```python
from build123d import *

# Parameters (mm, degrees)
SKETCH1_W                      = 20
SKETCH1_H                      = 8.2
BOSS_EXTRUDE1_DEPTH            = 21
SKETCH2_W                      = 8.2
SKETCH2_H                      = 0.8
BOSS_EXTRUDE2_DEPTH            = 5
SKETCH3_W                      = 8.2
SKETCH3_H                      = 0.8
BOSS_EXTRUDE3_DEPTH            = 5
CUT_EXTRUDE1_REACH             = 35.664
CUT_EXTRUDE2_REACH             = 33.217
F_2_0_2_DIAMETER_HOLE1_D       = 2
BOSS_EXTRUDE6_DEPTH            = 3
CUT_EXTRUDE4_REACH             = 36.986
SKETCH12_W                     = 6.2
SKETCH12_H                     = 2
BOSS_EXTRUDE7_DEPTH            = 3.5
BOSS_EXTRUDE7_TAPER            = 8
SKETCH15_R                     = 2
CUT_EXTRUDE5_DEPTH             = 5
SKETCH17_R                     = 3
SKETCH17_R_2                   = 2
BOSS_EXTRUDE10_DEPTH           = 0.2
BOSS_EXTRUDE10_DRAFT           = 45
SKETCH17_R_3                   = 1
BOSS_EXTRUDE10_PROFILE_2_DEPTH = 0.2
BOSS_EXTRUDE10_PROFILE_2_DRAFT = 45


with BuildPart() as part:
    # Sketch1 → Boss-Extrude1 (new body)
    with BuildSketch(Plane(origin=(0, 0, 0), x_dir=(1, 0, 0), z_dir=(0, 1, 0))):
        with Locations((10, -4.1)):
            Rectangle(SKETCH1_W, SKETCH1_H)
    extrude(amount=BOSS_EXTRUDE1_DEPTH)

    # Sketch2 → Boss-Extrude2 (add)
    with BuildSketch(Plane(origin=(20, 0, 0), x_dir=(0, 0, -1), z_dir=(1, 0, 0))):
        with Locations((-4.1, 16.4)):
            Rectangle(SKETCH2_W, SKETCH2_H)
    extrude(amount=BOSS_EXTRUDE2_DEPTH)

    # Sketch3 → Boss-Extrude3 (add)
    with BuildSketch(Plane.ZY):
        with Locations((4.1, 16.4)):
            Rectangle(SKETCH3_W, SKETCH3_H)
    extrude(amount=BOSS_EXTRUDE3_DEPTH)

    # Sketch4 → Cut-Extrude1 (cut, up to next)
    with BuildSketch(Plane.XY.offset(8.2), mode=Mode.PRIVATE) as cut_extrude1_sk1:
        Polygon((20, 19), (15, 21), (20, 21), align=None)
    cut_extrude1_tool1 = extrude(cut_extrude1_sk1.sketch, amount=-CUT_EXTRUDE1_REACH, mode=Mode.PRIVATE) & part.part
    add(cut_extrude1_tool1.solids().sort_by_distance((18.333333, 20.333333, 8.2))[0], mode=Mode.SUBTRACT)

    # Sketch8 → Cut-Extrude2 (cut, up to next)
    with BuildSketch(Plane(origin=(0, 16.8, 0), x_dir=(1, 0, 0), z_dir=(0, 1, 0)), mode=Mode.PRIVATE) as cut_extrude2_sk1:
        with BuildLine():
            Line((-5, 0), (0, 0))
            ThreePointArc((0, 0), (-4.1, -4.1), (0, -8.2))
            Line((0, -8.2), (-5, -8.2))
            Line((-5, -8.2), (-5, 0))
        make_face()
    cut_extrude2_tool1 = extrude(cut_extrude2_sk1.sketch, amount=-CUT_EXTRUDE2_REACH, mode=Mode.PRIVATE) & part.part
    # Sketch8 → Cut-Extrude2 (cut, up to next)
    with BuildSketch(Plane(origin=(0, 16.8, 0), x_dir=(1, 0, 0), z_dir=(0, 1, 0)), mode=Mode.PRIVATE) as cut_extrude2_sk2:
        with BuildLine():
            Line((20, -8.2), (25, -8.2))
            Line((25, -8.2), (25, 0))
            Line((25, 0), (20, 0))
            ThreePointArc((20, 0), (24.1, -4.1), (20, -8.2))
        make_face()
    cut_extrude2_tool2 = extrude(cut_extrude2_sk2.sketch, amount=-CUT_EXTRUDE2_REACH, mode=Mode.PRIVATE) & part.part
    add(cut_extrude2_tool1.solids().sort_by_distance((-2.5, 16.8, 8.103958))[0], mode=Mode.SUBTRACT)
    add(cut_extrude2_tool2.solids().sort_by_distance((24.196042, 16.8, 4.1))[0], mode=Mode.SUBTRACT)

    # Ø2.0 (2) Diameter Hole1 (through all)
    with Locations(Plane(origin=(-2.05, 16.8, 4.1), x_dir=(0, 0, 1), z_dir=(0, 1, 0))):
        with Locations((0, 0), (0, 24.1)):
            Hole(F_2_0_2_DIAMETER_HOLE1_D / 2)

    # Sketch10 → Boss-Extrude6 (add)
    with BuildSketch(Plane(origin=(0, 21, 0), x_dir=(1, 0, 0), z_dir=(0, 1, 0))):
        with BuildLine():
            ThreePointArc((7.886029412, -2.526474883), (0, -4.1), (7.886029412, -5.673525117))
            ThreePointArc((7.886029412, -5.673525117), (11.25, -4.1), (7.886029412, -2.526474883))
        make_face()
    extrude(amount=BOSS_EXTRUDE6_DEPTH)

    # Sketch11 → Cut-Extrude4 (cut, up to next)
    with BuildSketch(Plane.XY.offset(8.2), mode=Mode.PRIVATE) as cut_extrude4_sk1:
        Polygon((0, 0), (0, 2), (5, 0), align=None)
    cut_extrude4_tool1 = extrude(cut_extrude4_sk1.sketch, amount=-CUT_EXTRUDE4_REACH, mode=Mode.PRIVATE) & part.part
    add(cut_extrude4_tool1.solids().sort_by_distance((1.666667, 0.666667, 8.2))[0], mode=Mode.SUBTRACT)

    # Sketch12 → Boss-Extrude7 (add)
    with BuildSketch(Plane.ZY):
        with Locations((4.1, 8)):
            Rectangle(SKETCH12_W, SKETCH12_H)
    extrude(amount=BOSS_EXTRUDE7_DEPTH, taper=BOSS_EXTRUDE7_TAPER)

    # Sketch15 → Cut-Extrude5 (cut)
    with BuildSketch(Plane(origin=(0, 24, 0), x_dir=(1, 0, 0), z_dir=(0, 1, 0))):
        with Locations(Location((4.1, -4.1, 0), (0, 0, 270))):
            Circle(SKETCH15_R)
    extrude(amount=-CUT_EXTRUDE5_DEPTH, mode=Mode.SUBTRACT)


with BuildPart() as boss_extrude10_tool:
    # Sketch17 → Boss-Extrude10 (with draft: the straight prism first)
    with BuildSketch(Plane(origin=(0, 24, 0), x_dir=(1, 0, 0), z_dir=(0, 1, 0))):
        with Locations((4.1, -4.1)):
            Circle(SKETCH17_R)
        with Locations(Location((4.1, -4.1, 0), (0, 0, 270))):
            Circle(SKETCH17_R_2, mode=Mode.SUBTRACT)
    extrude(amount=BOSS_EXTRUDE10_DEPTH)
    # Boss-Extrude10: the draft: its side faces are tilted about the plane it starts from
    boss_extrude10_sides = [boss_extrude10_tool.faces().sort_by_distance(p)[0] for p in [
        (1.1, 24.1, 4.1),
        (4.1, 24.1, 2.1),
    ]]
    draft(boss_extrude10_sides, Plane(origin=(0, 24, 0), x_dir=(1, 0, 0), z_dir=(0, 1, 0)), BOSS_EXTRUDE10_DRAFT)


with BuildPart() as part_1:
    add(part.part)

    # Boss-Extrude10: add boss_extrude10_tool
    add(boss_extrude10_tool.part)


with BuildPart() as boss_extrude10_profile_2_tool:
    # Sketch17 → Boss-Extrude10 profile 2 (with draft: the straight prism first)
    with BuildSketch(Plane(origin=(0, 24, 0), x_dir=(1, 0, 0), z_dir=(0, 1, 0))):
        with Locations((9.2, -4.1)):
            Circle(SKETCH17_R_3)
    extrude(amount=BOSS_EXTRUDE10_PROFILE_2_DEPTH)
    # Boss-Extrude10 profile 2: the draft: its side faces are tilted about the plane it starts from
    boss_extrude10_profile_2_sides = [boss_extrude10_profile_2_tool.faces().sort_by_distance(p)[0] for p in [
        (8.2, 24.1, 4.1),
    ]]
    draft(boss_extrude10_profile_2_sides, Plane(origin=(0, 24, 0), x_dir=(1, 0, 0), z_dir=(0, 1, 0)), BOSS_EXTRUDE10_PROFILE_2_DRAFT)


with BuildPart() as part_2:
    add(part_1.part)

    # Boss-Extrude10 profile 2: add boss_extrude10_profile_2_tool
    add(boss_extrude10_profile_2_tool.part)


solid = part_2.part
```
Geometry check sheet. Reference: the model listing, model coordinates, mm. A direction names the side the tool comes from. Round coordinates to 2 decimals unless told otherwise and drop trailing zeros. Order: outer loops, then holes, each group sorted by start corner. A loop starts at its lowest first (then second) coordinate and runs counter-clockwise, first axis right, second up. Notation, with made-up numbers: M -14,81.5 L 33,81.5 A26 ccw 33,113.5 Z; hole C 89,-34 d9. An arc over 180 degrees is marked long. Write item = value, one per line.
Q1. Release check for a two-part mould opening along Z. For faces 4 (the flat face through (0.8, 21, 7.2)), 5 (the flat face through (10, 10, 0)), 6 (the flat face through (4, 19, 4)) record: released by +Z, released by -Z, zero draft, split by the parting line, or undercut.
Answer block:
face_4 = zero draft
face_5 = released by -Z
face_6 = undercut
Q2. Section check A-A (x = 9.2). Enter the section's corners in (y, z).
Answer block:
outline = M 0,0 L 21,0 L 21,2.05 L 24,2.05 L 24,3.1 L 24.2,3.3 L 24.2,4.9 L 24,5.1 L 24,6.15 L 21,6.15 L 21,8.2 L 0,8.2 Z
Q3. Set-up check for faces 1 (the flat face through (-0.7, 16, 4)), 2 (the flat face through (0, 19, 4)), 3 (the cylindrical face through (2.326, 21.535, 5.023)): record each of +Z, -Z, +X, -X, +Y, -Y from which the full face is reachable in a straight line by a thin tool's end or side.
Answer block:
face_1 = +Z, -Z, -X
face_2 = +Z, -Z, -X, +Y
face_3 = +Y
Q4. Section check C-C (z = 4.5). Give the number of separate pieces and of enclosed holes in the cut face, plus the area to 3 significant figures.
Answer block:
separate_pieces = 3
enclosed_holes = 0
area = 433 mm^2
Q5. Scan lines: line 1 (X direction, y = 16.35, z = 4.1); line 2 (X direction, y = 22.6, z = 4.1); line 3 (Y direction, x = 14, z = 7). Record each from-to range of solid material in increasing order.
Answer block:
line_1 = -4.1 to -3.05, -1.05 to 21.05, 23.05 to 24.1
line_2 = 0 to 2.1, 6.1 to 11.25
line_3 = 0 to 21
Q6. Depth check by flat-ended pin: pin 1 Ø1.2 at (x, z) = (22.5, 5.5) entering from +Y; pin 2 Ø3.5 at (x, z) = (-1, 4.5) entering from +Y; pin 3 Ø4 at (y, z) = (9.5, 6) entering from +X. Enter the tip coordinate at first touch or a pass-through.
Answer block:
pin_1 = 16.8
pin_2 = 24
pin_3 = 20
Q7. Section check B-B (z = 7.75). Enter the section's corners in (x, y).
Answer block:
outline = M -1.87,16 L 0,16 L 0,2 L 5,0 L 20,0 L 20,16 L 21.87,16 L 21.87,16.8 L 20,16.8 L 20,19 L 15,21 L 5.97,21 L 5.97,24 L 2.23,24 L 2.23,21 L 0,21 L 0,16.8 L -1.87,16.8 Z
